Part model, mm, in its own coordinate system. A direction names the side the tool comes from. Coordinates: 2 decimals unless noted, no trailing zeros. Order: outer loops, then holes, each group sorted by start corner. A loop starts at its lowest first (then second) coordinate and runs counter-clockwise, first axis right, second up. Notation, with made-up numbers: (-25.5, 57.5) - (-19.5, 57.5) arc R24 cw to (-19.5, 74.5) - close; hole circle Ø3 at (-39, 58). An arc over 180 degrees is marked (long way). Use a Markdown table: item, result. Add a question column.
1) Tool access for faces 4 (the face through (5.57, 4.37, 9.95)), 5 (the face through (7, -3, 0)), 6 (the face through (8.3, 6.04, 0.18)): list every direction of +Z, -Z, +X, -X, +Y, -Y with a clear straight run to the whole face (end or side of a thin tool).
2) Saw through at D-D on x = 3.5. List the corners of the cut face in (y, z).
3) Wall check: L1, parallel to Y at x = 5.25, z = -11.65; L2, parallel to Y at x = 10, z = -12.25; L3, parallel to Y at x = 1.5, z = 7. Give the ranges that are in metal, low to high. Write a range as [from, to].
4) Drop flat-ended pins along their axis: P1, Ø4, axis at x = 5.5, z = 1, coming from the +Y side; P2, Ø3, axis at y = 4.3, z = -11.65, coming from the +X side; P3, Ø6.5, axis at x = 3.5, z = -1.5, coming from the -Y side. Give the stop position or say it passes through.
5) Saw through at A-A on y = -3.5. List the corners of the cut face in (x, z), then the cut area to 3 significant figures.
6) Two-plate mould, pull along Y, no slides. Class faces 1 (the face through (5.57, -3.79, -10.03)), 2 (the face through (6, 0, -15)), 3 (the face through (9, 9, 0)): +Y half, -Y half, draft (parallel to the pull), parting line (faces both ways), or undercut.
7) Saw through at B-B on x = 10.5. List the corners of the cut face in (y, z).
8) Saw through at C-C on z = -11.65. List the corners of the cut face in (x, y).
```python
from build123d import *

# Parameters (mm, degrees)
SKETCH8_W           = 30
SKETCH8_H           = 100
BOSS_EXTRUDE1_DEPTH = 100
SKETCH9_W           = 88.7
SKETCH9_H           = 30
CUT_EXTRUDE1_DEPTH  = 103.708324882
SKETCH10_R          = 1.7
CUT_EXTRUDE2_DEPTH  = 21.825225089
FILLET1_R           = 1.5


with BuildPart() as part:
    # Sketch8 → Boss-Extrude1 (new body)
    with BuildSketch(Plane(origin=(0, 0, 0), x_dir=(0, 0, -1), z_dir=(1, 0, 0))):
        Rectangle(SKETCH8_W, SKETCH8_H)
    extrude(amount=BOSS_EXTRUDE1_DEPTH)

    # Sketch7 → Cut-Revolve3 (revolve, cut)
    with BuildSketch(Plane(origin=(0, 0, 0), x_dir=(0, 0, -1), z_dir=(1, 0, 0))):
        Polygon((-8.3, 9), (-150, 9), (-150, 50), (0, 50), (0, -50), (-150, -50), (-150, -9), (-8.3, -9), (-8.3, -3), (-6.3, -3), (-6.3, 3), (-8.3, 3), align=None)
    revolve(axis=Axis((0, -50, 0), (0, 1, 0)), mode=Mode.SUBTRACT)

    # Sketch9 → Cut-Extrude1 (cut, through all)
    with BuildSketch(Plane(origin=(0, 9, 0), x_dir=(1, 0, 0), z_dir=(0, 1, 0))):
        with Locations((55.65, 0)):
            Rectangle(SKETCH9_W, SKETCH9_H)
    extrude(amount=-CUT_EXTRUDE1_DEPTH, mode=Mode.SUBTRACT)

    # Sketch10 → Cut-Extrude2 (cut, through all)
    with BuildSketch(Plane.ZY):
        with Locations((-11.65, 4.3)):
            Circle(SKETCH10_R)
        with Locations((-11.65, -4.3)):
            Circle(SKETCH10_R)
        with Locations((11.65, -4.3)):
            Circle(SKETCH10_R)
        with Locations((11.65, 4.3)):
            Circle(SKETCH10_R)
    extrude(amount=-CUT_EXTRUDE2_DEPTH, mode=Mode.SUBTRACT)

    # Fillet1
    fillet1_edges = [part.edges().sort_by_distance(p)[0] for p in [
        (5.65, 9, 15),
        (5.65, -9, -15),
        (5.65, -9, 15),
        (5.65, 9, -15),
    ]]
    fillet(fillet1_edges, radius=FILLET1_R)


solid = part.part
```
Results are:
| question | item | result |
|---|---|---|
| 1 | face 4 | +X, -X |
| 1 | face 5 | -X, -Y |
| 1 | face 6 | -X, +Y |
| 2 | outline | (-9, -13.5) arc R1.5 ccw to (-7.5, -15) - (7.5, -15) arc R1.5 ccw to (9, -13.5) - (9, -7.53) - (3, -7.53) - (3, -5.24) - (-3, -5.24) - (-3, -7.53) - (-9, -7.53) - close; (-9, 7.53) - (-3, 7.53) - (-3, 5.24) - (3, 5.24) - (3, 7.53) - (9, 7.53) - (9, 13.5) arc R1.5 ccw to (7.5, 15) - (-7.5, 15) arc R1.5 ccw to (-9, 13.5) - close; hole circle Ø3.4 at (-4.3, -11.65); hole circle Ø3.4 at (-4.3, 11.65); hole circle Ø3.4 at (4.3, -11.65); hole circle Ø3.4 at (4.3, 11.65) |
| 3 | L1 | [-9, -6], [-2.6, 2.6], [6, 9] |
| 3 | L2 | [-9, -5.89], [-2.71, 2.71], [5.89, 9] |
| 3 | L3 | [-3, 3] |
| 4 | P1 | y = 3 |
| 4 | P2 | through |
| 4 | P3 | y = -3 |
| 5 | outline | (0, -15) - (11.3, -15) - (11.3, -13.15) - (0, -13.15) - close; (0, -10.15) - (11.3, -10.15) - (11.3, 10.15) - (0, 10.15) - (0, 8.3) arc R8.3 cw to (0, -8.3) - close; (0, 13.15) - (11.3, 13.15) - (11.3, 15) - (0, 15) - close |
| 5 | area | 163 mm2 |
| 6 | face 1 | undercut |
| 6 | face 2 | draft |
| 6 | face 3 | +Y half |
| 7 | outline | (-9, -13.5) arc R1.5 ccw to (-7.5, -15) - (7.5, -15) arc R1.5 ccw to (9, -13.5) - (9, 13.5) arc R1.5 ccw to (7.5, 15) - (-7.5, 15) arc R1.5 ccw to (-9, 13.5) - close; hole circle Ø3.4 at (-4.3, -11.65); hole circle Ø3.4 at (-4.3, 11.65); hole circle Ø3.4 at (4.3, -11.65); hole circle Ø3.4 at (4.3, 11.65) |
| 8 | outline | (0, -9) - (11.3, -9) - (11.3, -6) - (0, -6) - close; (0, -2.6) - (11.3, -2.6) - (11.3, 2.6) - (0, 2.6) - close; (0, 6) - (11.3, 6) - (11.3, 9) - (0, 9) - close |
